from build123d import *

# Parameters (mm, degrees)
SKETCH1_W           = 160
SKETCH1_H           = 30.4
BOSS_EXTRUDE1_DEPTH = 3.2
SKETCH2_W           = 160
SKETCH2_H           = 3.2
BOSS_EXTRUDE2_DEPTH = 4.8
SKETCH3_W           = 140.8
SKETCH3_H           = 16
CUT_EXTRUDE1_DEPTH  = 163.933115112
SKETCH4_W           = 9.6
SKETCH4_H           = 9.6
SKETCH4_R           = 1.5
BOSS_EXTRUDE3_DEPTH = 8


with BuildPart() as part:
    # Sketch1 → Boss-Extrude1 (new body)
    with BuildSketch(Plane(origin=(0, 0, 0), x_dir=(1, 0, 0), z_dir=(0, 1, 0))):
        with Locations((80, -15.2)):
            Rectangle(SKETCH1_W, SKETCH1_H)
    extrude(amount=BOSS_EXTRUDE1_DEPTH)

    # Sketch2 → Boss-Extrude2 (add)
    with BuildSketch(Plane(origin=(0, 3.2, 0), x_dir=(1, 0, 0), z_dir=(0, 1, 0))):
        with Locations((80, -28.8)):
            Rectangle(SKETCH2_W, SKETCH2_H)
        with Locations((80, -1.6)):
            Rectangle(SKETCH2_W, SKETCH2_H)
    extrude(amount=BOSS_EXTRUDE2_DEPTH)

    # Sketch3 → Cut-Extrude1 (cut, through all)
    with BuildSketch(Plane(origin=(0, 3.2, 0), x_dir=(1, 0, 0), z_dir=(0, 1, 0))):
        with Locations((80, -15.2)):
            Rectangle(SKETCH3_W, SKETCH3_H)
    extrude(amount=-CUT_EXTRUDE1_DEPTH, mode=Mode.SUBTRACT)

    # Sketch4 → Boss-Extrude3 (add)
    # profile 1 of 6: a face of its own
    with BuildSketch(Plane(origin=(0, 8, 0), x_dir=(1, 0, 0), z_dir=(0, 1, 0))):
        with Locations((28.8, -35.2)):
            Rectangle(SKETCH4_W, SKETCH4_H)
        with Locations(Location((28.8, -35.2, 0), (0, 0, 270))):
            Circle(SKETCH4_R, mode=Mode.SUBTRACT)
    # profile 2 of 6: a face of its own
    with BuildSketch(Plane(origin=(0, 8, 0), x_dir=(1, 0, 0), z_dir=(0, 1, 0))):
        with Locations((80, -35.2)):
            Rectangle(SKETCH4_W, SKETCH4_H)
        with Locations(Location((80, -35.2, 0), (0, 0, 270))):
            Circle(SKETCH4_R, mode=Mode.SUBTRACT)
    # profile 3 of 6: a face of its own
    with BuildSketch(Plane(origin=(0, 8, 0), x_dir=(1, 0, 0), z_dir=(0, 1, 0))):
        with Locations((131.2, -35.2)):
            Rectangle(SKETCH4_W, SKETCH4_H)
        with Locations(Location((131.2, -35.2, 0), (0, 0, 270))):
            Circle(SKETCH4_R, mode=Mode.SUBTRACT)
    # profile 4 of 6: a face of its own
    with BuildSketch(Plane(origin=(0, 8, 0), x_dir=(1, 0, 0), z_dir=(0, 1, 0))):
        with Locations((80, 4.8)):
            Rectangle(SKETCH4_W, SKETCH4_H)
        with Locations(Location((80, 4.8, 0), (0, 0, 270))):
            Circle(SKETCH4_R, mode=Mode.SUBTRACT)
    # profile 5 of 6: a face of its own
    with BuildSketch(Plane(origin=(0, 8, 0), x_dir=(1, 0, 0), z_dir=(0, 1, 0))):
        with Locations((131.2, 4.8)):
            Rectangle(SKETCH4_W, SKETCH4_H)
        with Locations(Location((131.2, 4.8, 0), (0, 0, 270))):
            Circle(SKETCH4_R, mode=Mode.SUBTRACT)
    # profile 6 of 6: a face of its own
    with BuildSketch(Plane(origin=(0, 8, 0), x_dir=(1, 0, 0), z_dir=(0, 1, 0))):
        with Locations((28.8, 4.8)):
            Rectangle(SKETCH4_W, SKETCH4_H)
        with Locations(Location((28.8, 4.8, 0), (0, 0, 270))):
            Circle(SKETCH4_R, mode=Mode.SUBTRACT)
    extrude(amount=-BOSS_EXTRUDE3_DEPTH)


solid = part.part
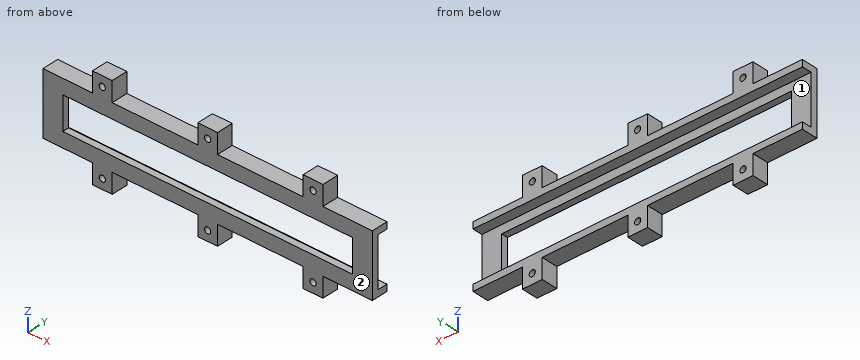
Model file for the job. Use its own axes, mm. Face numbers are marked on the shaded views. Round coordinates to 2 decimals unless told otherwise and drop trailing zeros. Order: outer loops, then holes, each group sorted by start corner. A loop starts at its lowest first (then second) coordinate and runs counter-clockwise, first axis right, second up.
(1) Band-saw the part on C-C (y = 5.5). Give the number of separate pieces and of enclosed holes in the cut face, then the cut area to 3 significant figures.
(2) Pull direction Z, two halves, no side cores. Call the marked faces 1 and 2: released by +Z, released by -Z, zero draft, split by the parting line, or undercut.
(3) Band-saw the part on D-D (z = 21). List the corners of the cut face in (x, y).
(4) Pin check, flat tips, straight feed: pin 1 (4 mm diameter, centred on y = 6, z = 33.5, fed in from -X); pin 2 (4 mm diameter, centred on x = 48, y = 4.5, fed in from -Z). Stop position of each tip, or through.
(5) Band-saw the part on B-B (x = 131.2). List the corners of the cut face in (y, z), then the cut area to 3 significant figures.
(6) Band-saw the part on A-A (z = 35.2). List the corners of the cut face in (x, y), then the cut area to 3 significant figures.
(7) Drill centre lines: line 1 (X direction, y = 5, z = -4.8); line 2 (X direction, y = 5.5, z = 33); line 3 (Z direction, x = 131.2, y = 3.25). Where is each one in solid material? Low to high.
Verdict:
1. separate pieces: 2
1. enclosed holes: 6
1. area: 1,530 mm2
2. face 1: undercut
2. face 2: zero draft
3. outline: (0, 0) - (9.6, 0) - (9.6, 3.2) - (0, 3.2) - close; (150.4, 0) - (160, 0) - (160, 3.2) - (150.4, 3.2) - close
4. pin 1: stops at x = 24
4. pin 2: stops at z = 0
5. outline: (0, -9.6) - (8, -9.6) - (8, -6.3) - (0, -6.3) - close; (0, -3.3) - (8, -3.3) - (8, 3.2) - (3.2, 3.2) - (3.2, 7.2) - (0, 7.2) - close; (0, 23.2) - (3.2, 23.2) - (3.2, 27.2) - (8, 27.2) - (8, 33.7) - (0, 33.7) - close; (0, 36.7) - (8, 36.7) - (8, 40) - (0, 40) - close
5. area: 182 mm2
6. outline: (24, 0) - (27.3, 0) - (27.3, 8) - (24, 8) - close; (30.3, 0) - (33.6, 0) - (33.6, 8) - (30.3, 8) - close; (75.2, 0) - (78.5, 0) - (78.5, 8) - (75.2, 8) - close; (81.5, 0) - (84.8, 0) - (84.8, 8) - (81.5, 8) - close; (126.4, 0) - (129.7, 0) - (129.7, 8) - (126.4, 8) - close; (132.7, 0) - (136, 0) - (136, 8) - (132.7, 8) - close
6. area: 158 mm2
7. line 1: x = 24 to 27.3, 30.3 to 33.6, 75.2 to 78.5, 81.5 to 84.8, 126.4 to 129.7, 132.7 to 136
7. line 2: x = 24 to 33.6, 75.2 to 84.8, 126.4 to 136
7. line 3: z = -9.6 to -6.3, -3.3 to 3.2, 27.2 to 33.7, 36.7 to 40
